The listing builds one solid part. Answer for the finished solid, in the listing's coordinates (mm). A direction names the side the tool comes from. Round coordinates to 2 decimals unless told otherwise and drop trailing zeros. Write each loop counter-clockwise with the first axis right and the second up, starting at its lowest first coordinate (ties: lowest second). Pieces come first, ordered by that corner, then holes.
from build123d import *

# Parameters (mm, degrees)
ESQUISSE1_W             = 68
ESQUISSE1_H             = 74
BOSS_EXTRU_1_DEPTH      = 34
ESQUISSE2_W             = 51
ESQUISSE2_H             = 21
ENL_V_MAT_EXTRU_1_DEPTH = 107.094297679
CHANFREIN1_SIZE         = 44
CHANFREIN1_SIZE2        = 20
CHANFREIN2_SIZE         = 44
CHANFREIN2_SIZE2        = 20
CHANFREIN3_SIZE         = 24
PER_AGE1_D              = 20
PER_AGE1_DEPTH          = 74
PER_AGE1_TIP            = 6.00860619


# Read off the part's stored shape, not the designer's step: Perçage2
with BuildPart() as part:
    # Esquisse1 → Boss.-Extru.1 (new, symmetric)
    with BuildSketch(Plane.XY):
        with Locations((34, 37)):
            Rectangle(ESQUISSE1_W, ESQUISSE1_H)
    extrude(amount=BOSS_EXTRU_1_DEPTH, both=True)

    # Esquisse2 → Enlèv. mat.-Extru.1 (cut, through all)
    with BuildSketch(Plane(origin=(68, 0, 0), x_dir=(0, 0, -1), z_dir=(1, 0, 0))):
        with Locations((-8.5, 22.5)):
            Rectangle(ESQUISSE2_W, ESQUISSE2_H)
    extrude(amount=-ENL_V_MAT_EXTRU_1_DEPTH, mode=Mode.SUBTRACT)

    # Chanfrein1
    chanfrein1_edges = [part.edges().sort_by_distance(p)[0] for p in [
        (68, 6, 34),
        (68, 53.5, 34),
    ]]
    chanfrein1_side = [part.faces().sort_by_distance(p)[0] for p in [
        (68, 40.920600858, -2.298283262),
    ]]
    chamfer(chanfrein1_edges, length=CHANFREIN1_SIZE, length2=CHANFREIN1_SIZE2, reference=chanfrein1_side[0])

    # Chanfrein2
    chanfrein2_edges = [part.edges().sort_by_distance(p)[0] for p in [
        (0, 6, 34),
        (0, 53.5, 34),
    ]]
    chanfrein2_side = [part.faces().sort_by_distance(p)[0] for p in [
        (0, 40.920600858, -2.298283262),
    ]]
    chamfer(chanfrein2_edges, length=CHANFREIN2_SIZE, length2=CHANFREIN2_SIZE2, reference=chanfrein2_side[0])

    # Chanfrein3
    chanfrein3_edges = [part.edges().sort_by_distance(p)[0] for p in [
        (34, 74, -34),
    ]]
    chamfer(chanfrein3_edges, length=CHANFREIN3_SIZE)

    # Perçage1
    with Locations(Plane(origin=(0, 74, 0), x_dir=(1, 0, 0), z_dir=(0, 1, 0))):
        with Locations((34, -14)):
            Hole(PER_AGE1_D / 2, depth=PER_AGE1_DEPTH)
            with Locations((0, 0, -(PER_AGE1_DEPTH + PER_AGE1_TIP / 2))):  # 118° drill point
                Cone(0, PER_AGE1_D / 2, PER_AGE1_TIP, mode=Mode.SUBTRACT)

    # Perçage2 outline → Perçage2 (revolve, cut)
    with BuildSketch(Plane(origin=(34, 61, 0), x_dir=(1, 0, 0), z_dir=(0, -1, 0))):
        Polygon((0, 23.682322777), (2.5, 23.682322777), (2.5, 33), (6, 33), (6, 34), (0, 34), align=None)
    revolve(axis=Axis((34, 61, 0), (0, 0, 1)), mode=Mode.SUBTRACT)


solid = part.part
1. A tool of negligible diameter and unlimited length cuts with its end or side. For faces 4 (the face through (0, 28, -22)), 5 (the face through (34, 12, 3)), 6 (the face through (33.46, 58.56, 28.4)), from which of +Z, -Z, +X, -X, +Y, -Y can it reach the whole face along a straight path? Write none if from no direction.
Geometry says:
face 4: +Z, -Z, -X, +Y, -Y
face 5: +Z, +X, -X
face 6: +Z
2. Section B-B on y = 7 is taken. Determine the outline of the cut face in (x, z), plus the area to 3 significant figures.
Geometry says:
outline: (0, -34) - (68, -34) - (68, -10) - (48, 34) - (20, 34) - (0, -10) - close; hole circle Ø20 at (34, 14)
area: 3,430 mm2
3. For a pull along X with two mould halves and no side action, classify faces 1 (the face through (58, 6, 12)), 2 (the face through (34, 22, -17)), 3 (the face through (34, 58, 33)) as released by +X, released by -X, zero draft, split by the parting line, or undercut.
Geometry says:
face 1: released by +X
face 2: zero draft
face 3: undercut
4. Section D-D on x = 7 is taken. Determine the outline of the cut face in (y, z).
Geometry says:
outline: (0, -34) - (50, -34) - (74, -10) - (74, 5.4) - (33, 5.4) - (33, -17) - (12, -17) - (12, 5.4) - (0, 5.4) - close
5. Section A-A on x = 34 is taken. Determine the outline of the cut face in (y, z).
Geometry says:
outline: (0, -34) - (50, -34) - (74, -10) - (74, 4) - (33, 4) - (33, -17) - (12, -17) - (12, 4) - (0, 4) - close; (0, 24) - (12, 24) - (12, 34) - (0, 34) - close; (33, 24) - (58.5, 24) - (58.5, 33) - (55, 33) - (55, 34) - (33, 34) - close; (63.5, 24) - (74, 24) - (74, 34) - (67, 34) - (67, 33) - (63.5, 33) - close
6. Straight lines are drawn through the part: line 1 along Y through (x, z) = (57.5, 0.5); line 2 along Z through (x, y) = (34, 3.5); line 3 along Y through (x, z) = (34, 33.4). For each, find the intervals that lie inside material, in ascending order.
Geometry says:
line 1: y = 0 to 12, 33 to 74
line 2: z = -34 to 4, 24 to 34
line 3: y = 0 to 12, 33 to 55, 67 to 74
7. Section C-C on z = 21 is taken. Determine the outline of the cut face in (x, y).
Geometry says:
outline: (14.09, 0) - (26.86, 0) - (26.86, 12) - (14.09, 12) - close; (14.09, 33) - (26.86, 33) - (26.86, 74) - (14.09, 74) - close; (41.14, 0) - (53.91, 0) - (53.91, 12) - (41.14, 12) - close; (41.14, 33) - (53.91, 33) - (53.91, 74) - (41.14, 74) - close
8. Given pin 1 (6 mm diameter, centred on y = 54, z = 18.5, fed in from +X); pin 2 (6 mm diameter, centred on y = 43.5, z = 19.5, fed in from -X); pin 3 (5 mm diameter, centred on y = 36.5, z = 27, fed in from -X), each flat-ended and moving along its own axis, determine where each tip first touches the part or whether it passes through.
Geometry says:
pin 1: stops at x = 56.41
pin 2: stops at x = 12.05
pin 3: stops at x = 15.68
